from build123d import *

# Parameters (mm, degrees)
SKETCH_1_W          = 31.99999989
SKETCH_1_H          = 11.5
SKETCH_1_R          = 2.2
EXTRUDE_1_DEPTH     = 29.5
SKETCH_2_R          = 2.5
CUT_EXTRUDE_1_DEPTH = 29.5


with BuildPart() as part:
    # 草图1 → 凸台-拉伸1 (new body)
    with BuildSketch(Plane.XY):
        with Locations((17.999999945, -43.99)):
            Rectangle(SKETCH_1_W, SKETCH_1_H)
        with Locations((8, -41.74)):
            Circle(SKETCH_1_R, mode=Mode.SUBTRACT)
        with Locations((27.99999989, -41.737899898)):
            Circle(SKETCH_1_R, mode=Mode.SUBTRACT)
    extrude(amount=EXTRUDE_1_DEPTH)

    # 草图2 → 切除-拉伸1 (cut)
    with BuildSketch(Plane.XZ.offset(49.74)):
        with Locations(Location((17.999999945, 14.75, 0), (0, 0, 270))):
            Circle(SKETCH_2_R)
    extrude(amount=-CUT_EXTRUDE_1_DEPTH, mode=Mode.SUBTRACT)


solid = part.part
Input: part model. Units: mm. Frame: model coordinates. Round coordinates to 2 decimals unless told otherwise and drop trailing zeros. Write each loop counter-clockwise with the first axis right and the second up, starting at its lowest first coordinate (ties: lowest second). Pieces come first, ordered by that corner, then holes.
1) Cut plane D-D (y = -48.5). Return the cut outline in (x, z), then the cut area to 3 significant figures.
2) Cut plane A-A (x = 28). Return the cut outline in (y, z), then the cut area to 3 significant figures.
3) Cut plane C-C (z = 14.75). Return the cut outline in (x, y), then the cut area to 3 significant figures.
4) Draft query along Y for faces 1 (the cylindrical face through (29.18, -39.88, 14.54)), 2 (the flat face through (18, -49.74, 11)), 3 (the flat face through (18, -38.24, 11)), 4 (the flat face through (18, -44, 29.5)). Return one class per face: pulls with the +Y half, pulls with the -Y half, needs draft (parallel to the pull), parting line crosses it, or undercut.
5) Cut plane B-B (y = -42.75). Return the cut outline in (x, z), then the cut area to 3 significant figures.
6) Ray query, L1, parallel to X at y = -41.75, z = 5.25; L2, parallel to X at y = -46, z = 14.75; L3, parallel to X at y = -42.75, z = 14.75. Return the intervals inside material, ascending.
Geometry says:
1. outline: (2, 0) - (34, 0) - (34, 29.5) - (2, 29.5) - close; hole circle Ø5 at (18, 14.75)
1. area: 924 mm2
2. outline: (-49.74, 0) - (-43.94, 0) - (-43.94, 29.5) - (-49.74, 29.5) - close; (-39.54, 0) - (-38.24, 0) - (-38.24, 29.5) - (-39.54, 29.5) - close
2. area: 209 mm2
3. outline: (2, -49.74) - (15.5, -49.74) - (15.5, -38.24) - (2, -38.24) - close; (20.5, -49.74) - (34, -49.74) - (34, -38.24) - (20.5, -38.24) - close; hole circle Ø4.4 at (8, -41.74); hole circle Ø4.4 at (28, -41.74)
3. area: 280 mm2
4. face 1: undercut
4. face 2: pulls with the -Y half
4. face 3: pulls with the +Y half
4. face 4: needs draft
5. outline: (2, 0) - (6.05, 0) - (6.05, 29.5) - (2, 29.5) - close; (9.95, 0) - (26.05, 0) - (26.05, 29.5) - (9.95, 29.5) - close; (29.95, 0) - (34, 0) - (34, 29.5) - (29.95, 29.5) - close; hole circle Ø5 at (18, 14.75)
5. area: 694 mm2
6. L1: x = 2 to 5.8, 10.2 to 25.8, 30.2 to 34
6. L2: x = 2 to 15.5, 20.5 to 34
6. L3: x = 2 to 6.05, 9.95 to 15.5, 20.5 to 26.05, 29.95 to 34
